The listing builds one solid part. Answer for the finished solid, in the listing's coordinates (mm). Round coordinates to 2 decimals unless told otherwise and drop trailing zeros. Loops run counter-clockwise (first coordinate to the right, second up) from the corner with the lowest first, then second, coordinate; pieces in that order, holes last. Notation, with made-up numbers: M 30.5,24 L 51.5,24 A27 cw 51.5,42 Z; hole C -4.5,-30 d4. An arc over 180 degrees is marked long. Put each result on its own line as item: value. Start each with the question number.
(1) Straight lines are drawn through the part: line 1 (Y direction, x = -36, z = 1.4); line 2 (X direction, y = -27, z = 2); line 3 (X direction, y = 2, z = 3.6). For each, find the intervals that lie inside material, in ascending order.
(2) Section B-B, the plane x = 0 is taken. Determine the outline of the cut face in (y, z), then the cut area to 3 significant figures.
(3) Section D-D, the plane z = 4.3 is taken. Count the separate pieces of the cut face and the enclosed holes in it, then the cut area to 3 significant figures.
(4) Section A-A, the plane y = 18 is taken. Determine the outline of the cut face in (x, z), then the cut area to 3 significant figures.
(5) Flat-ended cylindrical pins translate along their axes: P1, Ø9.5, axis at x = -30, y = 18, coming from the -Z side; P2, Ø2, axis at x = -9.5, y = -18, coming from the -Z side; P3, Ø2, axis at x = -26, z = 1, coming from the -Y side; P4, Ø3, axis at x = 25, z = 2.5, coming from the +Y side. Find the tip coordinate at first contact, or state that the pin passes through.
```python
from build123d import *

# Parameters (mm, degrees)
SKETCH2_R             = 40
SKETCH2_R_2           = 16
BOSS_EXTRUDE1_DEPTH   = 6
CUT_EXTRUDE1_DEPTH    = 3
M3X0_5_TAPPED_HOLE1_D = 2.5
CIRPATTERN1_COUNT     = 4
CHAMFER1_SIZE         = 1
HOLE1_D               = 3.4
HOLE1_CBORE_D         = 6.5
HOLE1_CBORE_DEPTH     = 3
CUT_EXTRUDE2_DEPTH    = 57.648036153
SKETCH11_W            = 8
SKETCH11_H            = 11
CUT_EXTRUDE3_DEPTH    = 57.885850613
FILLET1_R             = 2
FILLET2_R             = 2
CIRPATTERN2_DEPTH     = 6
M4_CLEARANCE_HOLE1_D  = 5
CIRPATTERN3_COUNT     = 4
FILLET3_R             = 2


# Read off the part's stored shape, not the designer's step: CirPattern2
with BuildPart() as part:
    # Sketch2 → Boss-Extrude1 (new body)
    with BuildSketch(Plane.XY):
        Circle(SKETCH2_R)
        Circle(SKETCH2_R_2, mode=Mode.SUBTRACT)
    extrude(amount=BOSS_EXTRUDE1_DEPTH)

    # Sketch3 → Cut-Extrude1 (cut)
    with BuildSketch(Plane(origin=(0, 0, 0), x_dir=(-1, 0, 0), z_dir=(0, 0, -1))):
        with BuildLine():
            Line((-8, 23.685438565), (-8, 41.112910233))
            ThreePointArc((-8, 41.112910233), (-29.61647673, 29.61647673), (-41.112910233, 8))
            Line((-41.112910233, 8), (-23.685438565, 8))
            ThreePointArc((-23.685438565, 8), (-17.67766953, 17.67766953), (-8, 23.685438565))
        make_face()
        with BuildLine():
            ThreePointArc((41.112910233, 8), (29.61647673, 29.61647673), (8, 41.112910233))
            Line((8, 41.112910233), (8, 23.685438565))
            ThreePointArc((8, 23.685438565), (17.67766953, 17.67766953), (23.685438565, 8))
            Line((23.685438565, 8), (41.112910233, 8))
        make_face()
        with BuildLine():
            Line((-23.685438565, -8), (-41.112910233, -8))
            ThreePointArc((-41.112910233, -8), (-29.61647673, -29.61647673), (-8, -41.112910233))
            Line((-8, -41.112910233), (-8, -23.685438565))
            ThreePointArc((-8, -23.685438565), (-17.67766953, -17.67766953), (-23.685438565, -8))
        make_face()
        with BuildLine():
            ThreePointArc((8, -41.112910233), (29.61647673, -29.61647673), (41.112910233, -8))
            Line((41.112910233, -8), (23.685438565, -8))
            ThreePointArc((23.685438565, -8), (17.67766953, -17.67766953), (8, -23.685438565))
            Line((8, -23.685438565), (8, -41.112910233))
        make_face()
    extrude(amount=-CUT_EXTRUDE1_DEPTH, mode=Mode.SUBTRACT)

    # M3x0.5 Tapped Hole1 (through all)
    with Locations(Plane(origin=(0, 0, 0), x_dir=(-1, 0, 0), z_dir=(0, 0, -1))):
        with Locations((-3.137606739, 35.863009131), (3.137606739, 35.863009131)):
            m3x0_5_tapped_hole1 = Hole(M3X0_5_TAPPED_HOLE1_D / 2)

    # CirPattern1: M3x0.5 Tapped Hole1 ×4 about axis
    cirpattern1_axis = Axis((0, 0, 0), (0, 0, 1))
    for i in range(1, CIRPATTERN1_COUNT):
        add(m3x0_5_tapped_hole1.rotate(cirpattern1_axis, i * 360 / CIRPATTERN1_COUNT), mode=Mode.SUBTRACT)

    # Chamfer1
    chamfer1_edges = [part.edges().sort_by_distance(p)[0] for p in [
        (-16, 0, 0),
    ]]
    chamfer(chamfer1_edges, length=CHAMFER1_SIZE)

    # Hole1 (through all)
    with Locations(Plane.XY.offset(6)):
        with Locations((-9.5, 18), (9.5, 18), (-9.5, -18), (9.5, -18)):
            CounterBoreHole(HOLE1_D / 2, HOLE1_CBORE_D / 2, HOLE1_CBORE_DEPTH)

    # Sketch10 → Cut-Extrude2 (cut, through all)
    with BuildSketch(Plane(origin=(0, 0, 3), x_dir=(-1, 0, 0), z_dir=(0, 0, -1))):
        with BuildLine():
            Line((-29.949958264, 8), (-23.685438565, 8))
            ThreePointArc((-23.685438565, 8), (-17.67766953, 17.67766953), (-8, 23.685438565))
            Line((-8, 23.685438565), (-8, 29.949958264))
            ThreePointArc((-8, 29.949958264), (-21.920310217, 21.920310217), (-29.949958264, 8))
        make_face()
    extrude(amount=-CUT_EXTRUDE2_DEPTH, mode=Mode.SUBTRACT)

    # Sketch11 → Cut-Extrude3 (cut, through all)
    with BuildSketch(Plane(origin=(0, 0, 0), x_dir=(-1, 0, 0), z_dir=(0, 0, -1))):
        with Locations((0, 26.5)):
            Rectangle(SKETCH11_W, SKETCH11_H)
    extrude(amount=-CUT_EXTRUDE3_DEPTH, mode=Mode.SUBTRACT)

    # Fillet1
    fillet1_edges = [part.edges().sort_by_distance(p)[0] for p in [
        (4, 21, 3),
        (4, 32, 3),
        (-4, 32, 3),
        (-4, 21, 3),
    ]]
    fillet(fillet1_edges, radius=FILLET1_R)

    # Fillet2
    fillet2_edges = [part.edges().sort_by_distance(p)[0] for p in [
        (8, 29.949958264, 4.5),
        (29.949958264, 8, 4.5),
        (8, 23.685438565, 3),
        (23.685438565, 8, 3),
    ]]
    fillet(fillet2_edges, radius=FILLET2_R)

    # CirPattern2 outline → CirPattern2 (cut)
    with BuildSketch(Plane.XY):
        with BuildLine():
            Line((-27.221315178, 8), (-23.685438565, 8))
            ThreePointArc((-23.685438565, 8), (-17.67766953, 17.67766953), (-8, 23.685438565))
            Line((-8, 23.685438565), (-8, 27.221315178))
            ThreePointArc((-8, 27.221315178), (-8.855297057, 28.861331998), (-10.689655172, 29.098647259))
            ThreePointArc((-10.689655172, 29.098647259), (-21.920310217, 21.920310217), (-29.098647259, 10.689655172))
            ThreePointArc((-29.098647259, 10.689655172), (-28.861331998, 8.855297057), (-27.221315178, 8))
        make_face()
        with BuildLine():
            Line((-8, -27.221315178), (-8, -23.685438565))
            ThreePointArc((-8, -23.685438565), (-17.67766953, -17.67766953), (-23.685438565, -8))
            Line((-23.685438565, -8), (-27.221315178, -8))
            ThreePointArc((-27.221315178, -8), (-28.861331998, -8.855297057), (-29.098647259, -10.689655172))
            ThreePointArc((-29.098647259, -10.689655172), (-21.920310217, -21.920310217), (-10.689655172, -29.098647259))
            ThreePointArc((-10.689655172, -29.098647259), (-8.855297057, -28.861331998), (-8, -27.221315178))
        make_face()
        with BuildLine():
            Line((27.221315178, -8), (23.685438565, -8))
            ThreePointArc((23.685438565, -8), (17.67766953, -17.67766953), (8, -23.685438565))
            Line((8, -23.685438565), (8, -27.221315178))
            ThreePointArc((8, -27.221315178), (8.855297057, -28.861331998), (10.689655172, -29.098647259))
            ThreePointArc((10.689655172, -29.098647259), (21.920310217, -21.920310217), (29.098647259, -10.689655172))
            ThreePointArc((29.098647259, -10.689655172), (28.861331998, -8.855297057), (27.221315178, -8))
        make_face()
        with BuildLine():
            ThreePointArc((2, -32), (3.414213562, -31.414213562), (4, -30))
            Line((4, -30), (4, -23))
            ThreePointArc((4, -23), (3.414213562, -21.585786438), (2, -21))
            Line((2, -21), (-2, -21))
            ThreePointArc((-2, -21), (-3.414213562, -21.585786438), (-4, -23))
            Line((-4, -23), (-4, -30))
            ThreePointArc((-4, -30), (-3.414213562, -31.414213562), (-2, -32))
            Line((-2, -32), (2, -32))
        make_face()
        with BuildLine():
            ThreePointArc((-21, 2), (-21.585786438, 3.414213562), (-23, 4))
            Line((-23, 4), (-30, 4))
            ThreePointArc((-30, 4), (-31.414213562, 3.414213562), (-32, 2))
            Line((-32, 2), (-32, -2))
            ThreePointArc((-32, -2), (-31.414213562, -3.414213562), (-30, -4))
            Line((-30, -4), (-23, -4))
            ThreePointArc((-23, -4), (-21.585786438, -3.414213562), (-21, -2))
            Line((-21, -2), (-21, 2))
        make_face()
        with BuildLine():
            ThreePointArc((32, 2), (31.414213562, 3.414213562), (30, 4))
            Line((30, 4), (23, 4))
            ThreePointArc((23, 4), (21.585786438, 3.414213562), (21, 2))
            Line((21, 2), (21, -2))
            ThreePointArc((21, -2), (21.585786438, -3.414213562), (23, -4))
            Line((23, -4), (30, -4))
            ThreePointArc((30, -4), (31.414213562, -3.414213562), (32, -2))
            Line((32, -2), (32, 2))
        make_face()
    extrude(amount=CIRPATTERN2_DEPTH, mode=Mode.SUBTRACT)

    # M4 Clearance Hole1 (through all)
    with Locations(Plane.XY.offset(6)):
        with Locations((-25.455844123, 25.455844123)):
            m4_clearance_hole1 = Hole(M4_CLEARANCE_HOLE1_D / 2)

    # CirPattern3: M4 Clearance Hole1 ×4 about axis
    cirpattern3_axis = Axis((0, 0, 0), (0, 0, 1))
    for i in range(1, CIRPATTERN3_COUNT):
        add(m4_clearance_hole1.rotate(cirpattern3_axis, i * 360 / CIRPATTERN3_COUNT), mode=Mode.SUBTRACT)

    # Fillet3
    fillet3_edges = [part.edges().sort_by_distance(p)[0] for p in [
        (23.685438565, -8, 1.5),
        (8, -23.685438565, 1.5),
        (-8, -23.685438565, 1.5),
        (-23.685438565, -8, 1.5),
        (-23.685438565, 8, 1.5),
        (-8, 23.685438565, 1.5),
    ]]
    fillet(fillet3_edges, radius=FILLET3_R)


solid = part.part
```
Recorded:
1. line 1: y = -8 to -4.38, -1.9 to 1.9, 4.38 to 8
1. line 2: x = -8 to -4, 4 to 8
1. line 3: x = -39.95 to -36.38, -35.34 to -32, -21 to -15.87, 15.87 to 21, 32 to 35.34, 36.38 to 39.95
2. outline: M -40,0 L -32,0 L -32,6 L -40,6 Z; M -21,0 L -17,0 L -16,1 L -16,6 L -21,6 Z; M 16,1 L 17,0 L 21,0 L 21,6 L 16,6 Z; M 32,0 L 40,0 L 40,6 L 32,6 Z
2. area: 155 mm²
3. separate pieces: 1
3. enclosed holes: 25
3. area: 2,980 mm²
4. outline: M -35.72,3 L -25.24,3 L -25.24,6 L -35.72,6 Z; M -17.35,0 L -11.2,0 L -11.2,3 L -12.75,3 L -12.75,6 L -17.35,6 Z; M -7.8,0 L 7.8,0 L 7.8,3 L 6.25,3 L 6.25,6 L -6.25,6 L -6.25,3 L -7.8,3 Z; M 11.2,0 L 17.35,0 L 17.35,6 L 12.75,6 L 12.75,3 L 11.2,3 Z; M 25.24,3 L 35.72,3 L 35.72,6 L 25.24,6 Z
4. area: 212 mm²
5. P1: stops at z = 3
5. P2: passes through
5. P3: stops at y = -8
5. P4: stops at y = 32.31
